```python
from build123d import *

# Parameters (mm, degrees)
SKETCH_1_W             = 140
SKETCH_1_H             = 31
SM_BASE_FLANGE_1_DEPTH = 6
OTHER_1_DEPTH          = 31
OTHER_1_2_DEPTH        = 31
SM_EDGE_FLANGE_1_DEPTH = 104.5
SKETCH_21_W            = 73.5
SKETCH_21_H            = 19
CUT_EXTRUDE_1_DEPTH    = 152.858486756
SKETCH_22_R            = 8
CUT_EXTRUDE_2_DEPTH    = 152.858486756
CHAMFER_1_SIZE         = 18
CHAMFER_1_SIZE2        = 31.176914536
FILLET_1_R             = 31


# Read off the part's stored shape, not the designer's step: 褶边1
# Sheet-metal steps are written as plain solids
with BuildPart() as part:
    # Sketch 1 → 基体-法兰1 (new body)
    with BuildSketch(Plane.XY):
        with Locations((-70, 15.5)):
            Rectangle(SKETCH_1_W, SKETCH_1_H)
    extrude(amount=-SM_BASE_FLANGE_1_DEPTH)

    # Other 1 outline → Other 1 (cut)
    with BuildSketch(Plane(origin=(0, 0, 0), x_dir=(1, 0, 0), z_dir=(0, 1, 0))):
        with BuildLine():
            ThreePointArc((-124.5, 0), (-131.319090848, 1.580589093), (-136.747448714, 6))
            Line((-136.747448714, 6), (-140, 6))
            Line((-140, 6), (-140, 0))
            Line((-140, 0), (-124.5, 0))
        make_face()
    extrude(amount=OTHER_1_DEPTH, mode=Mode.SUBTRACT)

    # Other 1 2 outline → Other 1 2 (add)
    with BuildSketch(Plane(origin=(0, 0, 0), x_dir=(1, 0, 0), z_dir=(0, 1, 0))):
        with BuildLine():
            Line((-20, 25), (-20, 31))
            Line((-20, 31), (-124.5, 31))
            ThreePointArc((-124.5, 31), (-138.419410907, 22.319090848), (-136.747448714, 6))
            Line((-136.747448714, 6), (-124.5, 6))
            ThreePointArc((-124.5, 6), (-134, 15.5), (-124.5, 25))
            Line((-124.5, 25), (-20, 25))
        make_face()
    extrude(amount=OTHER_1_2_DEPTH)

    # 边线-法兰1 section (across the edge) → 边线-法兰1 (add)
    with BuildSketch(Plane(origin=(-20, 44, -25), x_dir=(0, -1, 0), z_dir=(-1, 0, 0))):
        with BuildLine():
            Line((-6, 4), (-6, 25))
            Line((-6, 25), (0, 25))
            Line((0, 25), (0, 4))
            ThreePointArc((0, 4), (1.171572875, 1.171572875), (4, 0))
            Line((4, 0), (13, 0))
            Line((13, 0), (13, -6))
            Line((13, -6), (4, -6))
            ThreePointArc((4, -6), (-3.071067812, -3.071067812), (-6, 4))
        make_face()
    extrude(amount=SM_EDGE_FLANGE_1_DEPTH)

    # 草图21 → 切除-拉伸1 (cut, through all)
    with BuildSketch(Plane.XY):
        with Locations((-87.75, 40.5)):
            Rectangle(SKETCH_21_W, SKETCH_21_H)
    extrude(amount=-CUT_EXTRUDE_1_DEPTH, mode=Mode.SUBTRACT)

    # 草图22 → 切除-拉伸2 (cut, through all)
    with BuildSketch(Plane.XY):
        with Locations((-112, 16)):
            Circle(SKETCH_22_R)
        with Locations((-77, 16)):
            Circle(SKETCH_22_R)
    extrude(amount=-CUT_EXTRUDE_2_DEPTH, mode=Mode.SUBTRACT)

    # 倒角1
    chamfer_1_edges = [part.edges().sort_by_distance(p)[0] for p in [
        (0, 31, -3),
    ]]
    chamfer_1_side = [part.faces().sort_by_distance(p)[0] for p in [
        (0, 15.5, -3),
    ]]
    chamfer(chamfer_1_edges, length=CHAMFER_1_SIZE, length2=CHAMFER_1_SIZE2, reference=chamfer_1_side[0])

    # 圆角1
    fillet_1_edges = [part.edges().sort_by_distance(p)[0] for p in [
        (-20, 0, -28),
    ]]
    fillet(fillet_1_edges, radius=FILLET_1_R)


solid = part.part
```
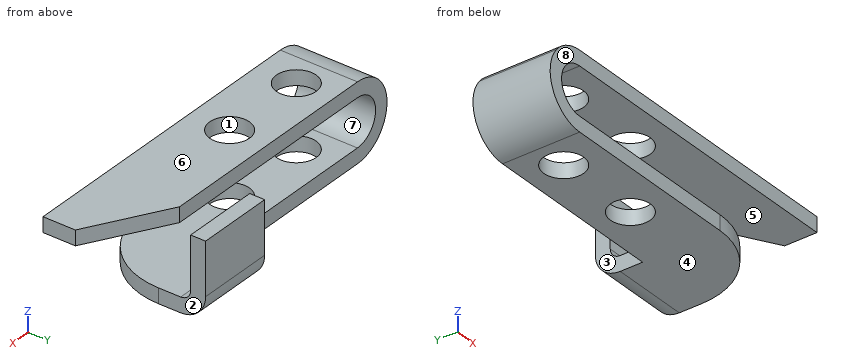
CAD build for the part. Positions are in the model's coordinates, mm. Face numbers are marked on the shaded views. A direction names the side the tool comes from. Give positions to 0.01 mm unless a question says otherwise; leave off trailing zeros. Loops run counter-clockwise (first coordinate to the right, second up) from the corner with the lowest first, then second, coordinate; pieces in that order, holes last. Notation, with made-up numbers: M 34,88 L 56,88 A28 cw 56,116 Z; hole C -12,-16.75 d10. An arc over 180 degrees is marked long. Use one line per item in the form item = value.
Item 1: Two-plate mould, pull along Z, no slides. Class the marked faces 6, 7 and 8: pulls with the +Z half, pulls with the -Z half, needs draft (parallel to the pull), parting line crosses it, or undercut.
Determined:
face_6 = pulls with the +Z half
face_7 = undercut
face_8 = needs draft
Item 2: Slice it at A-A (z = -15.5). List the corners of the cut face in (x, y).
Determined:
outline = M -140,0 L -134,0 L -134,31 L -140,31 Z; M -51,44 L -20,44 L -20,50 L -51,50 Z
Item 3: Slice it at D-D (z = -9.5). List the corners of the cut face in (x, y), plus the area to 3 significant figures.
Determined:
outline = M -138.79,0 L -131.87,0 L -131.87,31 L -138.79,31 Z; M -51,44 L -20,44 L -20,50 L -51,50 Z
area = 401 mm2
Item 4: Drill centre lines: probe 1 along Z at (x, y) = (-53.5, 8); probe 2 along Y at (x, z) = (-77, -26.5); probe 3 along X at (y, z) = (9.5, -27.5). Where is each one in solid material? Low to high. Write a range as from..to.
Determined:
probe_1 = -31..-25, -6..0
probe_2 = 0..8, 24..31
probe_3 = -134.31..-116.66, -107.34..-81.66, -72.34..-28.67
Item 5: Flat gauge pins, fed straight in: pin 1 (18.5 mm diameter, centred on x = -77, y = 16, fed in from +Z); pin 2 (6 mm diameter, centred on y = 25.5, z = -26.5, fed in from +X); pin 3 (6 mm diameter, centred on y = 10, z = -21, fed in from -X); pin 4 (6.5 mm diameter, centred on x = -41.5, z = -11, fed in from -Y). Where does each tip first touch, or does it go through?
Determined:
pin_1 = 0
pin_2 = -20.1
pin_3 = -139.8
pin_4 = 44
Item 6: Which spindle directions (+Z, -Z, +X, -X, +Y, -Y) get a long thin tool onto all of the face, cutting with end or side? Do the marked faces 1, 2, 3, 4 and 5. Say none if no direction does.
Determined:
face_1 = +Z, -Z
face_2 = +Z, -Z, +X, +Y
face_3 = +Z, -Z, -X, +Y
face_4 = -Z, +X, -X, +Y, -Y
face_5 = +X, -Y
Item 7: Slice it at C-C (y = 16). List the corners of the cut face in (x, z).
Determined:
outline = M -124.5,-31 L -120,-31 L -120,-25 L -124.5,-25 A9.5 cw -124.5,-6 L -120,-6 L -120,0 L -124.5,0 A15.5 ccw Z; M -104,-31 L -85,-31 L -85,-25 L -104,-25 Z; M -104,-6 L -85,-6 L -85,0 L -104,0 Z; M -69,-31 L -23.87,-31 L -23.87,-25 L -69,-25 Z; M -69,-6 L -5.2,-6 L -5.2,0 L -69,0 Z
Item 8: Slice it at B-B (x = -112). List the corners of the cut face in (y, z), plus the area to 3 significant figures.
Determined:
outline = M 0,-31 L 8,-31 L 8,-25 L 0,-25 Z; M 0,-6 L 8,-6 L 8,0 L 0,0 Z; M 24,-31 L 31,-31 L 31,-25 L 24,-25 Z; M 24,-6 L 31,-6 L 31,0 L 24,0 Z
area = 180 mm2
